Check sheet for the drawn part. Datum: minimum x, y, z corner. Units: mm. A direction names the side the tool comes from. Round coordinates to 2 decimals unless told otherwise and drop trailing zeros. Write each loop counter-clockwise with the first axis right and the second up, starting at its lowest first coordinate (ties: lowest second). Pieces come first, ordered by that corner, then holes. Notation, with made-up numbers: M 48,78 L 65,78 A25 cw 65,113 Z; hole C 65.25,50 d11. An arc over 180 degrees is marked long. Put each result on its own line as item: value.
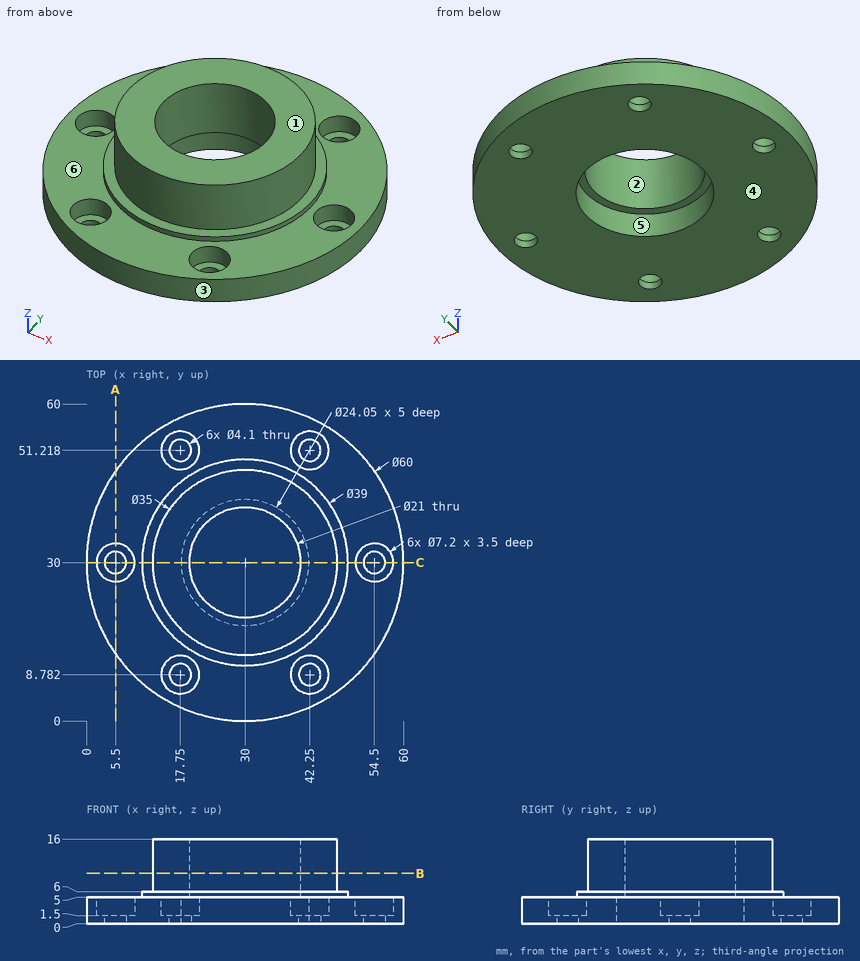
1. Depth check by flat-ended pin: pin 1 Ø4 at (x, y) = (28, 12.5) entering from +Z; pin 2 Ø10 at (x, y) = (46, 53.5) entering from +Z; pin 3 Ø8 at (x, z) = (38, 5.5) entering from +Y; pin 4 Ø3 at (y, z) = (40, 9.5) entering from -X. Enter the tip coordinate at first touch or a pass-through.
Computed values:
pin 1: stops at z = 16
pin 2: stops at z = 5
pin 3: stops at y = 59.73
pin 4: stops at x = 14.7
2. Cross-section at B-B (z = 9.5). Enter the section's corners in (x, y).
Computed values:
outline: C 30,30 d35; hole C 30,30 d21
3. Cross-section at C-C (y = 30). Count the separate pieces of the cut face and the enclosed holes in it, then the cut area to 3 significant figures.
Computed values:
separate pieces: 4
enclosed holes: 0
area: 275 mm2
4. Cross-section at A-A (x = 5.5). Enter the section's corners in (y, z).
Computed values:
outline: M 12.69,0 L 27.95,0 L 27.95,1.5 L 26.4,1.5 L 26.4,5 L 12.69,5 Z; M 32.05,0 L 47.31,0 L 47.31,5 L 33.6,5 L 33.6,1.5 L 32.05,1.5 Z
5. Release check for a two-part mould opening along Y. For the marked faces 1, 2 and 3 record: +Y half, -Y half, draft (parallel to the pull), parting line (faces both ways), or undercut.
Computed values:
face 1: draft
face 2: undercut
face 3: parting line
6. Access from +Z, -Z, +X, -X, +Y, -Y to the whole of each face (thin tool, end or side, straight path). Record for the marked faces 4, 5 and 6.
Computed values:
face 4: -Z, +X, -X, +Y, -Y
face 5: -Z
face 6: +Z
7. Scan lines: probe 1 along Y at (x, z) = (17.75, 0.85) (1 decimal); probe 2 along Z at (x, y) = (52.5, 40); probe 3 along X at (y, z) = (26, 8.75). Record each from-to range of solid material in increasing order.
Computed values:
probe 1: y = 2.6 to 6.7, 10.8 to 49.2, 53.3 to 57.4
probe 2: z = 0 to 5
probe 3: x = 12.96 to 20.29, 39.71 to 47.04
